Could you check a few things on this model? Use its own coordinates, in mm. Face numbers are marked on the shaded views. Coordinates: 2 decimals unless noted, no trailing zeros. Order: outer loops, then holes, each group sorted by start corner. A loop starts at its lowest first (then second) coordinate and runs counter-clockwise, first axis right, second up.
Autodesk Inventor part; units mm, degrees
ref_plane "YZ Plane" through (0, 0, 0) normal (1, 0, 0) x (0, 1, 0)
ref_plane "XZ Plane" through (0, 0, 0) normal (0, 1, 0) x (-1, 0, 0)
ref_plane "XY Plane" through (0, 0, 0) normal (0, 0, 1) x (1, 0, 0)
sketch "Esboço1" plane through (0, 0, 0) normal (0, 0, 1) x (1, 0, 0)
  line L0 (0, 0) -> (50, 0)
  line L1 (50, 0) -> (50, 10)
  line L2 (0, 0) -> (0, 30)
  line L3 (0, 30) -> (20, 30)
  line L4 (20, 30) -> (50, 10)
  dimension "d0" = 50
  dimension "d1" = 10
  dimension "d2" = 30
  dimension "d3" = 20
extrude "Extrusão1" add sketch "Esboço1" along normal blind 10
sketch "Esboço2" plane through (0, 0, 10) normal (0, 0, 1) x (1, 0, 0)
  line L0 (0, 30) -> (0, 0)
  line L1 (0, 0) -> (50, 0)
  point P0 (15, 15)
  dimension "d6" = 15
  dimension "d14" = 15
hole "Furo1" at (15, 15, 10) direction (0, 0, -1) diameter 10 end through all
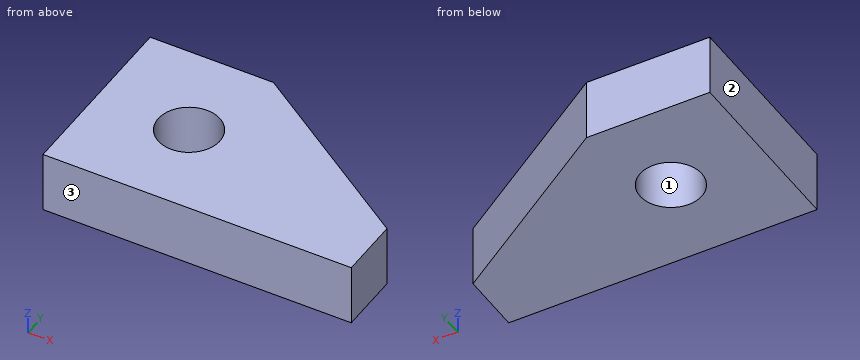
Item 1: Suppose I cut it at A-A (y = 18). List the corners of the cut face in (x, z) for me.
Item 2: Suppose I cut it at C-C (z = 5). List the corners of the cut face in (x, y) for me, and give its area (3 significant figures).
Item 3: Suppose I cut it at B-B (x = 15). List the corners of the cut face in (y, z) for me, and give its area (3 significant figures).
Item 4: Suppose I cut it at D-D (y = 28). List the corners of the cut face in (x, z) for me.
Item 5: For pin 1 Ø5 at (x, y) = (29.5, 3) entering from -Z; pin 2 Ø4 at (y, z) = (25, 3) entering from +X, each with a flat end and sliding along its axis, tell me the tip position at first contact or that it passes through.
Item 6: Thinking about a two-plate mould opening in Y: for the marked faces 1, 2 and 3, which applies, +Y half, -Y half, draft (parallel to the pull), parting line (faces both ways), or undercut?
Item 7: I need wall thicknesses on line 1 (Y direction, x = 15, z = 6.5); line 2 (X direction, y = 13.5, z = 4.75); line 3 (X direction, y = 18, z = 5). Which ranges of each line are inside material? Lowest first, please.
Geometry results:
1. outline: (0, 0) - (11, 0) - (11, 10) - (0, 10) - close; (19, 0) - (38, 0) - (38, 10) - (19, 10) - close
2. outline: (0, 0) - (50, 0) - (50, 10) - (20, 30) - (0, 30) - close; hole circle Ø10 at (15, 15)
2. area: 1,120 mm2
3. outline: (0, 0) - (10, 0) - (10, 10) - (0, 10) - close; (20, 0) - (30, 0) - (30, 10) - (20, 10) - close
3. area: 200 mm2
4. outline: (0, 0) - (23, 0) - (23, 10) - (0, 10) - close
5. pin 1: stops at z = 0
5. pin 2: stops at x = 30.5
6. face 1: undercut
6. face 2: draft
6. face 3: -Y half
7. line 1: y = 0 to 10, 20 to 30
7. line 2: x = 0 to 10.23, 19.77 to 44.75
7. line 3: x = 0 to 11, 19 to 38
